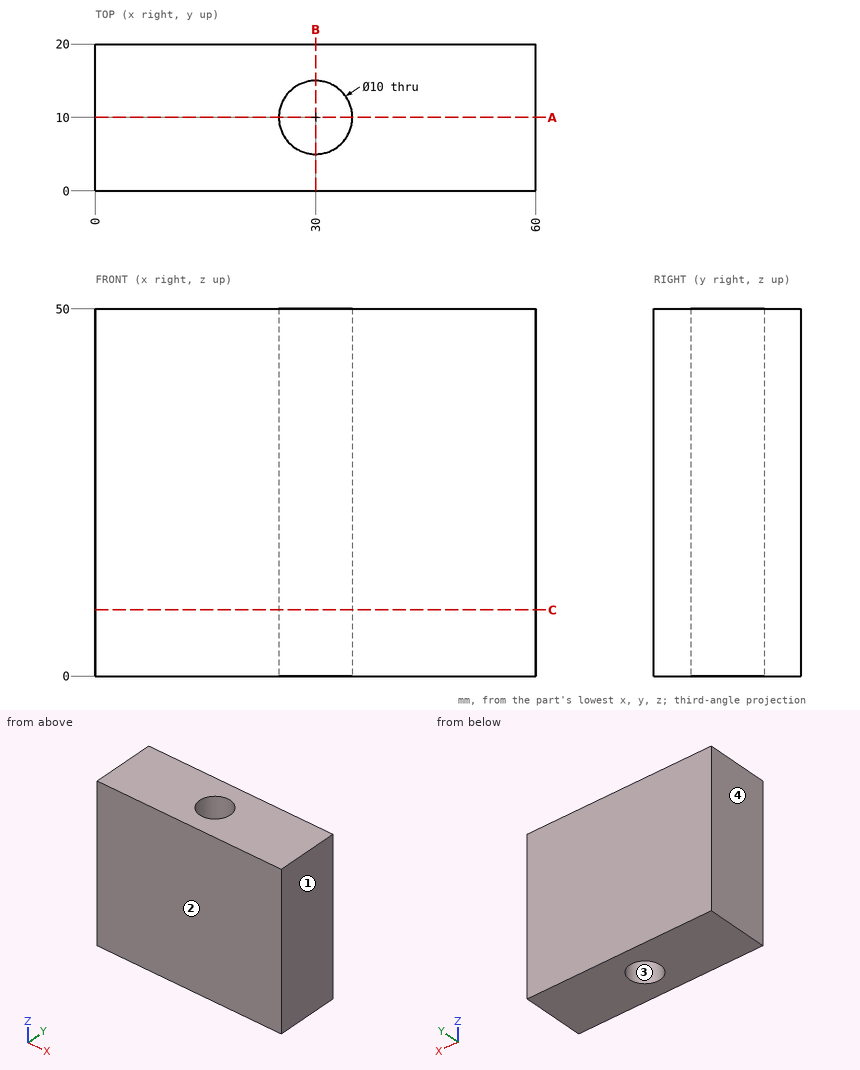
Answer from the drawing. Dimensions are ordinates in mm from the lowest x, y and z of the part. Give positions to 0.01 mm unless a question says otherwise; leave off trailing zeros. Order: outer loops, then holes, each group sorted by start corner. A loop starts at its lowest first (then second) coordinate and runs counter-clockwise, first axis right, second up. Notation, with made-up numbers: (-36, 8) - (22, 8) arc R6 ccw to (22, 14) - close; hole circle Ø4 at (61.5, 16.5). An arc over 180 degrees is marked (long way). Use one line per item in the form item = value.
1) The mould has two halves that part along X. Classify the marked faces 1, 2, 3 and 4: released by +X, released by -X, zero draft, split by the parting line, or undercut.
Verdict:
face_1 = released by +X
face_2 = zero draft
face_3 = undercut
face_4 = released by -X
2) Find section B-B on x = 30. Determine the outline of the cut face in (y, z).
Verdict:
outline = (0, 0) - (5, 0) - (5, 50) - (0, 50) - close; (15, 0) - (20, 0) - (20, 50) - (15, 50) - close
3) Find section A-A on y = 10. Determine the outline of the cut face in (x, z), and give its area (3 significant figures).
Verdict:
outline = (0, 0) - (25, 0) - (25, 50) - (0, 50) - close; (35, 0) - (60, 0) - (60, 50) - (35, 50) - close
area = 2,500 mm^2
4) Find section C-C on z = 9. Determine the outline of the cut face in (x, y), and give its area (3 significant figures).
Verdict:
outline = (0, 0) - (60, 0) - (60, 20) - (0, 20) - close; hole circle Ø10 at (30, 10)
area = 1,120 mm^2
5) Consider probe 1 along Y at (x, z) = (30, 29); probe 2 along X at (y, z) = (9.75, 26.5); probe 3 along Y at (x, z) = (26.5, 21.5). Determine where each line is inside the solid, lowest interval first. Write a range as [from, to].
Verdict:
probe_1 = [0, 5], [15, 20]
probe_2 = [0, 25.01], [34.99, 60]
probe_3 = [0, 6.43], [13.57, 20]
